from build123d import *

# Parameters (mm, degrees)
F0_R     = 8.375
F1_DEPTH = 12.5
F2_R     = 6.375
F3_DEPTH = 10
F4_R     = 1.404945
F5_DEPTH = 75


with BuildPart() as f1:
    # F0 (on Top) → F1 (new body)
    with BuildSketch(Plane.XY):
        with Locations((19.557578, 38.052302)):
            Circle(F0_R)
    extrude(amount=F1_DEPTH)

    # F2 (on face) → F3 (cut)
    with BuildSketch(Plane.XY.offset(12.5)):
        with Locations((19.557578, 38.052302)):
            Circle(F2_R)
    extrude(amount=-F3_DEPTH, mode=Mode.SUBTRACT)

    # F4 (on Front) → F5 (cut)
    with BuildSketch(Plane.XZ):
        with Locations((19.41436, 10.001411)):
            Circle(F4_R)
    extrude(amount=-F5_DEPTH, mode=Mode.SUBTRACT)


solid = f1.part
CAD build for the part. Positions are in the model's coordinates, mm. Round coordinates to 2 decimals unless told otherwise and drop trailing zeros. Write each loop counter-clockwise with the first axis right and the second up, starting at its lowest first coordinate (ties: lowest second). Pieces come first, ordered by that corner, then holes.
(1) Slice it at B-B, the plane y = 42.5. Write the cut outline in (x, z).
(2) Slice it at C-C, the plane x = 21.5. Write the cut outline in (y, z), and give its area (3 significant figures).
(3) Mould opens along Y. For faces 1 (the face through (22.499, 32.397, 7.57)), 2 (the face through (20.754, 45.316, 10.423)), 3 (the face through (19, 38, 2.5)), 4 (the face through (17.742, 29.876, 6.162)) say: pulls with the +Y half, pulls with the -Y half, needs draft (parallel to the pull), parting line crosses it, or undercut.
(4) Probe line 1 along Z through (x, y) = (21.5, 43.5); line 2 along Y through (x, z) = (19, 3.75); line 3 along X through (y, z) = (37.25, 8.5). List the from-to ranges inside material, lowest first.
(5) Slice it at D-D, the plane z = 4. Write the cut outline in (x, y) (3 decimals), and give its area (3 significant figures).
(6) Drop flat-ended pins along their axis: P1, Ø10, axis at x = 19.56, y = 38.05, coming from the +Z side; P2, Ø1.7, axis at x = 19.41, z = 10, coming from the +Y side; P3, Ø1.5, axis at y = 44.5, z = 7.5, coming from the -X side; P4, Ø5, axis at x = 16.5, z = 7.5, coming from the -Y side. Give the stop position or say it passes through.
(7) Slice it at A-A, the plane x = 18.25. Write the cut outline in (y, z).
From the geometry:
1. outline: (12.46, 0) - (26.65, 0) - (26.65, 12.5) - (24.12, 12.5) - (24.12, 2.5) - (14.99, 2.5) - (14.99, 12.5) - (12.46, 12.5) - close
2. outline: (29.91, 0) - (46.2, 0) - (46.2, 12.5) - (44.12, 12.5) - (44.12, 2.5) - (31.98, 2.5) - (31.98, 12.5) - (29.91, 12.5) - close
2. area: 82.2 mm2
3. face 1: undercut
3. face 2: needs draft
3. face 3: undercut
3. face 4: parting line crosses it
4. line 1: z = 0 to 2.5
4. line 2: y = 29.7 to 31.7, 44.4 to 46.41
4. line 3: x = 11.22 to 13.23, 25.88 to 27.89
5. outline: circle Ø16.75 at (19.558, 38.052); hole circle Ø12.75 at (19.558, 38.052)
5. area: 92.7 mm2
6. P1: stops at z = 2.5
6. P2: passes through
6. P3: stops at x = 13.42
6. P4: stops at y = 29.7
7. outline: (29.78, 0) - (46.32, 0) - (46.32, 9.22) - (44.29, 9.22) - (44.29, 2.5) - (31.81, 2.5) - (31.81, 9.22) - (29.78, 9.22) - close; (29.78, 10.79) - (31.81, 10.79) - (31.81, 12.5) - (29.78, 12.5) - close; (44.29, 10.79) - (46.32, 10.79) - (46.32, 12.5) - (44.29, 12.5) - close
